CAD build for the part. Positions are in the model's coordinates, mm. A direction names the side the tool comes from. Round coordinates to 2 decimals unless told otherwise and drop trailing zeros. Order: outer loops, then holes, each group sorted by start corner. A loop starts at its lowest first (then second) coordinate and runs counter-clockwise, first axis right, second up. Notation, with made-up numbers: M 40.5,3 L 86.5,3 A32 cw 86.5,42 Z; hole C 45.25,-31.5 d5. An arc over 180 degrees is marked long. Answer as a JSON object with one key per item and string values.
```python
from build123d import *

# Parameters (mm, degrees)
SKETCH2_W           = 571.5
SKETCH2_H           = 139.7
BOSS_EXTRUDE2_DEPTH = 38.1
SKETCH3_W           = 88.9
SKETCH3_H           = 50.8
CUT_EXTRUDE1_DEPTH  = 590.559114933
SKETCH4_R           = 41.275
CUT_EXTRUDE2_DEPTH  = 590.559114933
SKETCH5_R           = 4.7625
CUT_EXTRUDE3_DEPTH  = 580.626664328
SKETCH6_R           = 4.7625
CUT_EXTRUDE4_DEPTH  = 580.626664328
SKETCH7_W           = 101.6
SKETCH7_H           = 6.35
CUT_EXTRUDE5_DEPTH  = 590.559114933


with BuildPart() as part:
    # Sketch2 → Boss-Extrude2 (new body)
    with BuildSketch(Plane.XY):
        with Locations((285.75, 69.85)):
            Rectangle(SKETCH2_W, SKETCH2_H)
    extrude(amount=BOSS_EXTRUDE2_DEPTH)

    # Sketch3 → Cut-Extrude1 (cut, through all)
    with BuildSketch(Plane.XY.offset(38.1)):
        with Locations((44.45, 114.3)):
            Rectangle(SKETCH3_W, SKETCH3_H)
        with Locations((527.05, 114.3)):
            Rectangle(SKETCH3_W, SKETCH3_H)
        with Locations((527.05, 25.4)):
            Rectangle(SKETCH3_W, SKETCH3_H)
        with Locations((44.45, 25.4)):
            Rectangle(SKETCH3_W, SKETCH3_H)
    extrude(amount=-CUT_EXTRUDE1_DEPTH, mode=Mode.SUBTRACT)

    # Sketch4 → Cut-Extrude2 (cut, through all)
    with BuildSketch(Plane.XY.offset(38.1)):
        with Locations((381.247583626, 69.85)):
            Circle(SKETCH4_R)
    extrude(amount=-CUT_EXTRUDE2_DEPTH, mode=Mode.SUBTRACT)

    # Sketch5 → Cut-Extrude3 (cut, through all)
    with BuildSketch(Plane(origin=(0, 50.8, 0), x_dir=(-1, 0, 0), z_dir=(0, -1, 0))):
        with Locations(Location((-44.45, -19.05, 0), (0, 0, 180))):
            Circle(SKETCH5_R)
    extrude(amount=-CUT_EXTRUDE3_DEPTH, mode=Mode.SUBTRACT)

    # Sketch6 → Cut-Extrude4 (cut, through all)
    with BuildSketch(Plane.XZ.offset(-50.8)):
        with Locations((527.05, 19.05)):
            Circle(SKETCH6_R)
    extrude(amount=-CUT_EXTRUDE4_DEPTH, mode=Mode.SUBTRACT)

    # Sketch7 → Cut-Extrude5 (cut, through all)
    with BuildSketch(Plane.XZ):
        with Locations((381, 3.175)):
            Rectangle(SKETCH7_W, SKETCH7_H)
    extrude(amount=-CUT_EXTRUDE5_DEPTH, mode=Mode.SUBTRACT)


solid = part.part
```
Item 1: Saw through at D-D on y = 14.5. List the corners of the cut face in (x, z).
Worked answers:
{"outline": "M 88.9,0 L 330.2,0 L 330.2,6.35 L 431.8,6.35 L 431.8,0 L 482.6,0 L 482.6,38.1 L 88.9,38.1 Z"}
Item 2: Wall check: line 1 along X through (y, z) = (67, 19); line 2 along X through (y, z) = (116, 6); line 3 along X through (y, z) = (69, 30). Give the ranges that are in metal, low to high. Write a range as [from, to].
Worked answers:
{"line 1": "x = [0, 39.69], [49.21, 340.07], [422.42, 522.29], [531.81, 571.5]", "line 2": "x = [88.9, 330.2], [431.8, 482.6]", "line 3": "x = [0, 339.98], [422.51, 571.5]"}
Item 3: Two-plate mould, pull along X, no slides. Class faces 1 (the flat face through (482.6, 25, 19)), 2 (the cylindrical face through (522.292, 69.583, 19.259)), 3 (the flat face through (44, 50.8, 28)): released by +X, released by -X, zero draft, split by the parting line, or undercut.
Worked answers:
{"face 1": "released by +X", "face 2": "undercut", "face 3": "zero draft"}
Item 4: Drop flat-ended pins along their axis: pin 1 Ø4 at (y, z) = (41.5, 33.5) entering from +X; pin 2 Ø19 at (x, z) = (49.5, 23) entering from +Y; pin 3 Ø2 at (x, z) = (487, 20) entering from -Y; pin 4 Ø7.5 at (x, z) = (44.45, 19.05) entering from +Y. Give the stop position or say it passes through.
Worked answers:
{"pin 1": "stops at x = 482.6", "pin 2": "stops at y = 88.9", "pin 3": "stops at y = 50.8", "pin 4": "passes through"}
Item 5: Saw through at B-B on x = 44.45. List the corners of the cut face in (y, z).
Worked answers:
{"outline": "M 50.8,0 L 88.9,0 L 88.9,14.29 L 50.8,14.29 Z; M 50.8,23.81 L 88.9,23.81 L 88.9,38.1 L 50.8,38.1 Z"}
Item 6: 3-axis set-ups, long thin cutter, end or side, ignore diameter. For faces 4 (the flat face through (88.9, 114, 19)), 5 (the flat face through (425, 69, 6.35)), 6 (the flat face through (283, 0, 19)), 7 (the flat face through (526, 50.8, 28)), 8 (the flat face through (482.6, 114, 19)): which of +Z, -Z, +X, -X, +Y, -Y reach the whole face in a straight line?
Worked answers:
{"face 4": "+Z, -Z, -X, +Y", "face 5": "-Z, +Y, -Y", "face 6": "+Z, -Z, +X, -X, -Y", "face 7": "+Z, -Z, +X, -Y", "face 8": "+Z, -Z, +X, +Y"}
Item 7: Saw through at A-A on z = 19.05. State how many separate pieces and enclosed holes the cut face has, and give its area (3 significant figures).
Worked answers:
{"separate pieces": "3", "enclosed holes": "1", "area": "55,700 mm2"}
